from build123d import *

# Parameters (mm, degrees)
SKETCH1_W           = 20
SKETCH1_H           = 9
BOSS_EXTRUDE1_DEPTH = 3
SKETCH2_R           = 1.35
CUT_EXTRUDE1_DEPTH  = 12.368817001
SKETCH3_R           = 2.5
CUT_EXTRUDE2_DEPTH  = 2
SKETCH4_W           = 6
SKETCH4_H           = 9
BOSS_EXTRUDE2_DEPTH = 20
SKETCH7_W           = 3
SKETCH7_H           = 9
BOSS_EXTRUDE5_DEPTH = 7
SKETCH8_W           = 9
SKETCH8_H           = 9
BOSS_EXTRUDE6_DEPTH = 4
CHAMFER1_SIZE       = 4
SKETCH9_R           = 2.05
CUT_EXTRUDE3_DEPTH  = 32.941352507


with BuildPart() as part:
    # Sketch1 → Boss-Extrude1 (new body)
    with BuildSketch(Plane(origin=(0, 0, 0), x_dir=(1, 0, 0), z_dir=(0, 1, 0))):
        Rectangle(SKETCH1_W, SKETCH1_H)
    extrude(amount=BOSS_EXTRUDE1_DEPTH)

    # Sketch2 → Cut-Extrude1 (cut, through all)
    with BuildSketch(Plane(origin=(0, 3, 0), x_dir=(1, 0, 0), z_dir=(0, 1, 0))):
        with Locations(Location((-6, 0, 0), (0, 0, 270))):
            Circle(SKETCH2_R)
        with Locations(Location((6, 0, 0), (0, 0, 270))):
            Circle(SKETCH2_R)
    extrude(amount=-CUT_EXTRUDE1_DEPTH, mode=Mode.SUBTRACT)

    # Sketch3 → Cut-Extrude2 (cut)
    with BuildSketch(Plane(origin=(0, 3, 0), x_dir=(1, 0, 0), z_dir=(0, 1, 0))):
        with Locations(Location((-6, 0, 0), (0, 0, 270))):
            Circle(SKETCH3_R)
        with Locations(Location((6, 0, 0), (0, 0, 270))):
            Circle(SKETCH3_R)
    extrude(amount=-CUT_EXTRUDE2_DEPTH, mode=Mode.SUBTRACT)

    # Sketch4 → Boss-Extrude2 (add)
    with BuildSketch(Plane(origin=(0, 3, 0), x_dir=(1, 0, 0), z_dir=(0, 1, 0))):
        Rectangle(SKETCH4_W, SKETCH4_H)
    extrude(amount=BOSS_EXTRUDE2_DEPTH)

    # Sketch7 → Boss-Extrude5 (add)
    with BuildSketch(Plane(origin=(0, 23, 0), x_dir=(1, 0, 0), z_dir=(0, 1, 0))):
        with Locations((1.5, 0)):
            Rectangle(SKETCH7_W, SKETCH7_H)
    extrude(amount=BOSS_EXTRUDE5_DEPTH)

    # Sketch8 → Boss-Extrude6 (add)
    with BuildSketch(Plane(origin=(3, 0, 0), x_dir=(0, 0, -1), z_dir=(1, 0, 0))):
        with Locations((0, 25.5)):
            Rectangle(SKETCH8_W, SKETCH8_H)
    extrude(amount=BOSS_EXTRUDE6_DEPTH)

    # Chamfer1
    chamfer1_edges = [part.edges().sort_by_distance(p)[0] for p in [
        (3, 21, 0),
    ]]
    chamfer(chamfer1_edges, length=CHAMFER1_SIZE - 0.0001)  # a hair under: the kernel refuses the full size

    # Sketch9 → Cut-Extrude3 (cut, through all)
    with BuildSketch(Plane.ZY):
        with Locations((0, 26.5)):
            Circle(SKETCH9_R)
    extrude(amount=-CUT_EXTRUDE3_DEPTH, mode=Mode.SUBTRACT)


solid = part.part
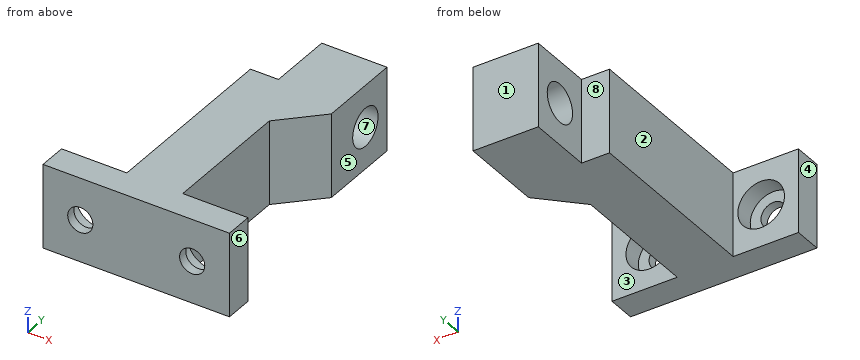
Can you work these out from the model? Positions are in its coordinate system, mm. Face numbers are marked on the shaded views. A direction names the side the tool comes from. Give positions to 0.01 mm unless a question says otherwise; leave off trailing zeros. Loops run counter-clockwise (first coordinate to the right, second up) from the corner with the lowest first, then second, coordinate; pieces in that order, holes last. Notation, with made-up numbers: (17.5, -11.75) - (65.5, -11.75) arc R24 ccw to (65.5, 6.25) - close; hole circle Ø8 at (43.5, 79). An arc over 180 degrees is marked (long way). Return JSON: item names as keys, results as strings.
1. I want a section at A-A on z = 0. Give the number of separate pieces and of enclosed holes in the cut face, and give its area (3 significant figures).
Output values:
{"separate pieces": "4", "enclosed holes": "0", "area": "191 mm²"}
2. I want a section at B-B on y = 26.5. Please give me the cut outline in (x, z).
Output values:
{"outline": "(0, -4.5) - (7, -4.5) - (7, -2.05) - (0, -2.05) - close; (0, 2.05) - (7, 2.05) - (7, 4.5) - (0, 4.5) - close"}
3. If I drill on line 1 (X direction, y = 0.5, z = 0); line 2 (Y direction, x = 4.5, z = 0); line 3 (X direction, y = 2, z = 2), over which ranges is the centre line in solid material (lowest first)?
Output values:
{"line 1": "x = -10 to -7.35, -4.65 to 4.65, 7.35 to 10", "line 2": "y = 0 to 1, 18.5 to 24.45, 28.55 to 30", "line 3": "x = -10 to -7.5, -4.5 to 4.5, 7.5 to 10"}
4. We'd pull the mould along Y, two halves only. Please class the marked faces 6, 7 and 8: +Y half, -Y half, draft (parallel to the pull), parting line (faces both ways), or undercut.
Output values:
{"face 6": "draft", "face 7": "undercut", "face 8": "+Y half"}
5. For the marked faces 1, 2, 3, 4 and 5, which set-ups out of +Z, -Z, +X, -X, +Y, -Y let a thin tool reach every point of the face, with its end or its side?
Output values:
{"face 1": "+Z, -Z, +X, -X, +Y", "face 2": "+Z, -Z, -X, +Y", "face 3": "+Z, -Z, +X", "face 4": "+Z, -Z, -X, +Y, -Y", "face 5": "+Z, -Z, +X, +Y"}
6. I'm going to push flat-ended pins straight in: pin 1 Ø5 at (y, z) = (6.5, 0) entering from +X; pin 2 Ø4 at (x, z) = (-6, 0) entering from +Y; pin 3 Ø4.5 at (y, z) = (26.5, 0) entering from +X. Where does each tip first touch, or does it pass through?
Output values:
{"pin 1": "stops at x = 3", "pin 2": "stops at y = 1", "pin 3": "stops at x = 7"}
7. I want a section at C-C on x = 6. Please give me the cut outline in (y, z).
Output values:
{"outline": "(0, -4.5) - (3, -4.5) - (3, -2.5) - (1, -2.5) - (1, -1.35) - (0, -1.35) - close; (0, 1.35) - (1, 1.35) - (1, 2.5) - (3, 2.5) - (3, 4.5) - (0, 4.5) - close; (20, -4.5) - (30, -4.5) - (30, 4.5) - (20, 4.5) - close; hole circle Ø4.1 at (26.5, 0)"}
